Geometry check sheet. Reference: the model listing, model coordinates, mm. Face numbers are marked on the shaded views. A direction names the side the tool comes from. Coordinates: 2 decimals unless noted, no trailing zeros. Order: outer loops, then holes, each group sorted by start corner. A loop starts at its lowest first (then second) coordinate and runs counter-clockwise, first axis right, second up. Notation, with made-up numbers: M 58.25,-0.75 L 90.25,-0.75 A16 ccw 90.25,10.25 Z; hole C -18,-29 d3. An arc over 180 degrees is marked long. One line per item, written item: value. Start each with the question number.
1) Sectioned sample at C-C, the plane x = 12.5. Enter the section's corners in (y, z) (3 decimals).
2) Sectioned sample at D-D, the plane x = 29.5. Enter the section's corners in (y, z) (3 decimals).
3) Access from +Z, -Z, +X, -X, +Y, -Y to the whole of each face (thin tool, end or side, straight path). Record for the marked faces 4, 5, 6 and 7.
4) Go/stop test with flat-tipped pins: P1, Ø6, axis at x = 26.5, y = 11.5, coming from the -Z side; P2, Ø22, axis at x = 48, y = 29, coming from the +Z side (3 decimals); P3, Ø5, axis at x = 43, z = 19, coming from the -Y side; P4, Ø17.5, axis at y = 17, z = 7, coming from the -X side. Record where each tip stops, or that it passes through.
5) Sectioned sample at A-A, the plane z = 20.5. Enter the section's corners in (x, y).
6) Thickness scan on L1, parallel to Y at x = 50.5, z = 2 (3 decimals); L2, parallel to Y at x = 7, z = 10.5; L3, parallel to Z at x = 33, y = 10.5 (3 decimals). Record the ranges inside material, lowest first. Write a range as from..to.
7) Draft check along Z on the marked faces 1, 2 and 3. Enter one of: pulls with the +Z half, pulls with the -Z half, needs draft (parallel to the pull), parting line crosses it, or undercut.
8) Sectioned sample at B-B, the plane y = 37.5. Enter the section's corners in (x, z) (3 decimals), then the cut area to 3 significant figures.
```python
from build123d import *

# Parameters (mm, degrees)
F0_W     = 76.2
F0_H     = 44.45
F1_DEPTH = 33.02
F2_W     = 57.15
F2_H     = 44.45
F3_DEPTH = 17.145
F4_W     = 26.67
F4_H     = 3.175
F5_DEPTH = 19.05
F6_W     = 34.29
F6_H     = 12.7
F7_DEPTH = 10.16


with BuildPart() as f1:
    # F0 (on Top) → F1 (new body)
    with BuildSketch(Plane.XY):
        with Locations((38.1, 22.225)):
            Rectangle(F0_W, F0_H)
    extrude(amount=F1_DEPTH)

    # F2 (on face) → F3 (cut)
    with BuildSketch(Plane.XY.offset(33.02)):
        with Locations((47.625, 22.225)):
            Rectangle(F2_W, F2_H)
    extrude(amount=-F3_DEPTH, mode=Mode.SUBTRACT)

    # F4 (on face) → F5 (cut)
    with BuildSketch(Plane(origin=(0, 0, 0), x_dir=(0, -1, 0), z_dir=(-1, 0, 0))):
        Polygon((-35.56, 29.845), (-40.64, 29.845), (-40.64, 3.175), (-35.56, 3.175), (-8.89, 3.175), (-3.81, 3.175), (-3.81, 29.845), (-8.89, 29.845), align=None)
        with Locations((-22.225, 31.4325)):
            Rectangle(F4_W, F4_H)
        with Locations((-22.225, 1.5875)):
            Rectangle(F4_W, F4_H)
    extrude(amount=-F5_DEPTH, mode=Mode.SUBTRACT)

    # F6 (on face) → F7 (cut)
    with BuildSketch(Plane(origin=(0, 0, 0), x_dir=(1, 0, 0), z_dir=(0, 0, -1))):
        with BuildLine():
            ThreePointArc((53.34, -28.575), (59.69, -22.225), (53.34, -15.875))
            Line((53.34, -15.875), (53.34, -28.575))
        make_face()
        with Locations((36.195, -22.225)):
            Rectangle(F6_W, F6_H)
    extrude(amount=-F7_DEPTH, mode=Mode.SUBTRACT)


solid = f1.part
```
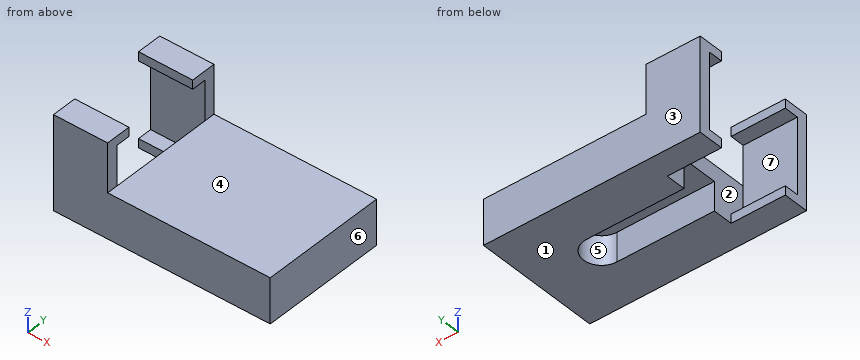
Final values:
1. outline: M 0,0 L 8.89,0 L 8.89,3.175 L 3.81,3.175 L 3.81,29.845 L 8.89,29.845 L 8.89,33.02 L 0,33.02 Z; M 35.56,0 L 44.45,0 L 44.45,33.02 L 35.56,33.02 L 35.56,29.845 L 40.64,29.845 L 40.64,3.175 L 35.56,3.175 Z
2. outline: M 0,0 L 15.875,0 L 15.875,10.16 L 28.575,10.16 L 28.575,0 L 44.45,0 L 44.45,15.875 L 0,15.875 Z
3. face 4: +Z, +X, +Y, -Y
3. face 5: -Z, -X
3. face 6: +Z, -Z, +X, +Y, -Y
3. face 7: -X
4. P1: stops at z = 0
4. P2: stops at z = 15.875
4. P3: passes through
4. P4: stops at x = 19.05
5. outline: M 0,0 L 19.05,0 L 19.05,3.81 L 0,3.81 Z; M 0,40.64 L 19.05,40.64 L 19.05,44.45 L 0,44.45 Z
6. L1: y = 0..15.875, 28.575..44.45
6. L2: y = 0..3.81, 40.64..44.45
6. L3: z = 0..15.875
7. face 1: pulls with the -Z half
7. face 2: undercut
7. face 3: needs draft
8. outline: M 0,0 L 76.2,0 L 76.2,15.875 L 19.05,15.875 L 19.05,3.175 L 0,3.175 Z; M 0,29.845 L 19.05,29.845 L 19.05,33.02 L 0,33.02 Z
8. area: 1,030 mm^2
